For this review, use the dimensioned drawing (mm, ordinates from the lowest corner) and the shaded views. A direction names the side the tool comes from. Coordinates: 2 decimals unless noted, no trailing zeros. Loops run counter-clockwise (first coordinate to the right, second up) from the corner with the lowest first, then second, coordinate; pieces in that order, holes last. Notation, with made-up numbers: M -7.75,-35 L 25.25,-35 A21 ccw 25.25,0 Z; hole C 28.25,-8.75 d7. An arc over 180 degrees is marked long. One line per item, written item: value.
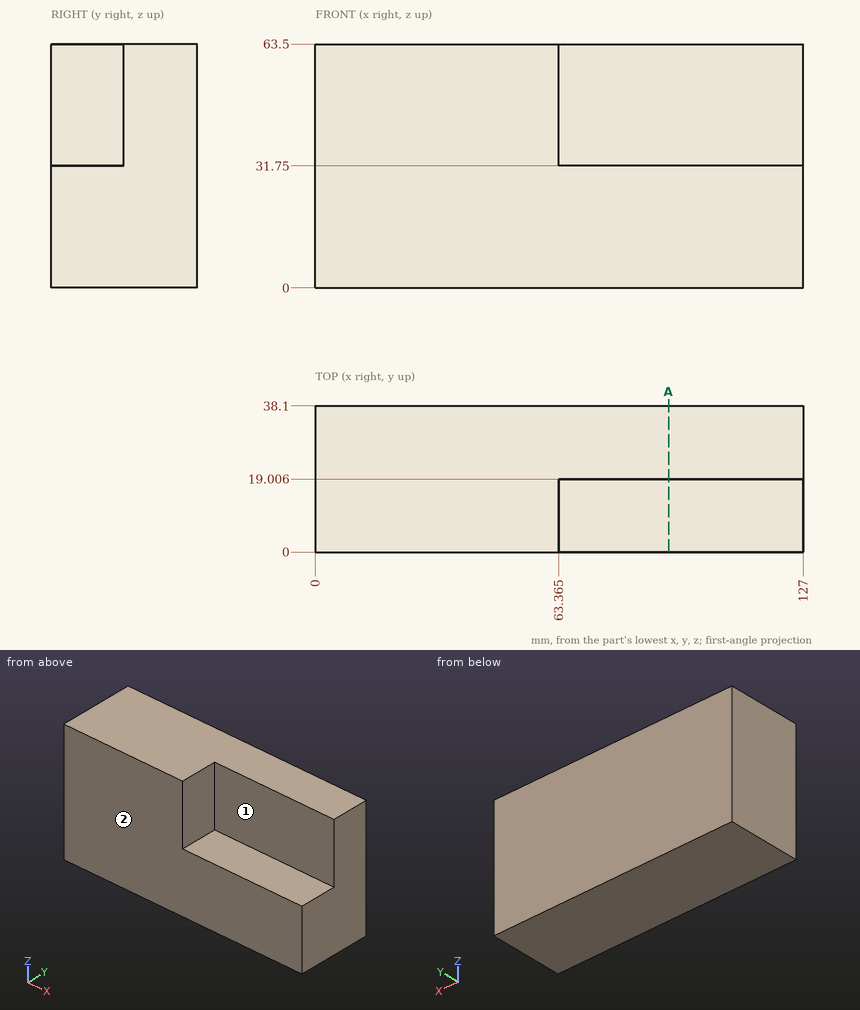
(1) To check wall thickness, follow L1, parallel to Y at x = 68.5, z = 54; L2, parallel to Z at x = 88, y = 14; L3, parallel to X at y = 8, z = 35.5 (1 decimal). State the ranges of each line that lie inside material, in increasing order. Write a range as [from, to].
Checks:
L1: [19.01, 38.1]
L2: [0, 31.75]
L3: [0, 63.4]
(2) Tool access review of the marked faces 1 and 2: name each direction out of +Z, -Z, +X, -X, +Y, -Y from which nothing blocks a thin tool from reaching the whole face with its end or side.
Checks:
face 1: +Z, +X, -Y
face 2: +Z, -Z, +X, -X, -Y
(3) Add section A-A on x = 92. State the section outline as (y, z) points, then the cut area to 3 significant figures.
Checks:
outline: M 0,0 L 38.1,0 L 38.1,63.5 L 19.01,63.5 L 19.01,31.75 L 0,31.75 Z
area: 1,820 mm^2
(4) Insertion check: pin 1 Ø4 at (x, z) = (58.5, 54) entering from -Y; pin 2 Ø15 at (x, y) = (95.5, 6) entering from +Z; pin 3 Ø1 at (y, z) = (6.5, 56) entering from +X (1 decimal). Each pin has a flat end and moves straight along its axis. Give the tip position at first contact, or say it passes through.
Checks:
pin 1: y = 0
pin 2: z = 31.75
pin 3: x = 63.4
